Design review of the part built by this model. Coordinates are the model's own, in mm. Face numbers are marked on the shaded views. Round coordinates to 2 decimals unless told otherwise and drop trailing zeros. Order: outer loops, then holes, each group sorted by start corner. A loop starts at its lowest first (then second) coordinate and runs counter-clockwise, first axis right, second up. Notation, with made-up numbers: (17.25, 31) - (51.25, 31) arc R15 ccw to (51.25, 48) - close; hole circle Ø10 at (70, 68). An arc over 180 degrees is marked (long way). Use CSV: the item, a comma, the result in double quotes.
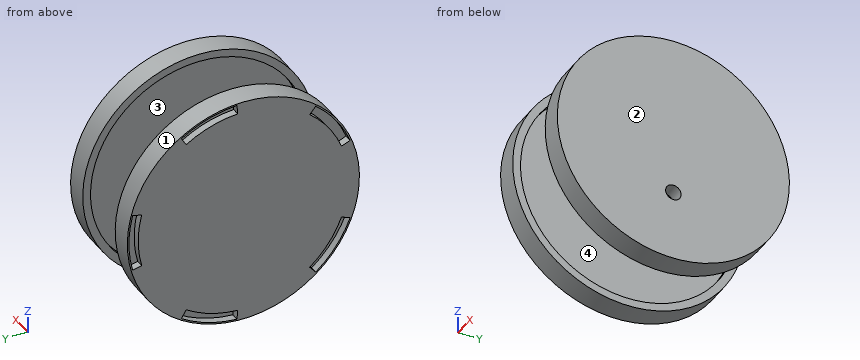
from build123d import *

# Parameters (mm, degrees)
CUT_EXTRUDE1_DEPTH = 5
CIRPATTERN1_COUNT  = 5
SKETCH4_R          = 5
CUT_EXTRUDE4_DEPTH = 16


with BuildPart() as part:
    # Sketch1 → Revolve2 (revolve)
    with BuildSketch(Plane.XY, mode=Mode.PRIVATE) as revolve2_sk:
        Polygon((-52.115384615, 0), (17.884615385, 0), (17.884615385, 75), (2.884615385, 75), (2.884615385, 70), (7.884615385, 70), (7.884615385, 20), (-42.115384615, 20), (-42.115384615, 70), (-37.115384615, 70), (-37.115384615, 75), (-52.115384615, 75), align=None)
    revolve(revolve2_sk.sketch.rotate(Axis((-114.1965821, 0, 0), (1, 0, 0)), 90), axis=Axis((-114.1965821, 0, 0), (1, 0, 0)))

    # Sketch2 → Cut-Extrude1 (cut)
    with BuildSketch(Plane.ZY.offset(52.115384615)):
        with BuildLine():
            Line((-18.889553649, 71.548478411), (-17.514771122, 65.705652668))
            ThreePointArc((-17.514771122, 65.705652668), (0, 68), (17.514771122, 65.705652668))
            Line((17.514771122, 65.705652668), (18.889553649, 71.548478411))
            ThreePointArc((18.889553649, 71.548478411), (0, 74), (-18.889553649, 71.548478411))
        make_face()
    cut_extrude1 = extrude(amount=-CUT_EXTRUDE1_DEPTH, mode=Mode.SUBTRACT)

    # CirPattern1: Cut-Extrude1 ×5 about axis
    cirpattern1_axis = Axis((0, 0, 0), (1, 0, 0))
    for i in range(1, CIRPATTERN1_COUNT):
        add(cut_extrude1.rotate(cirpattern1_axis, i * 360 / CIRPATTERN1_COUNT), mode=Mode.SUBTRACT)

    # Sketch4 → Cut-Extrude4 (cut)
    with BuildSketch(Plane(origin=(17.884615385, 0, 0), x_dir=(0, 0, -1), z_dir=(1, 0, 0))):
        with Locations((29.519700861, 0)):
            Circle(SKETCH4_R)
    extrude(amount=-CUT_EXTRUDE4_DEPTH, mode=Mode.SUBTRACT)


solid = part.part
1) The part is to be moulded in two halves that separate along Z. For the marked faces 1, 2, 3 and 4, say which applies: +Z half, -Z half, draft (parallel to the pull), parting line (faces both ways), or undercut.
Data:
face 1,"parting line"
face 2,"draft"
face 3,"undercut"
face 4,"undercut"
2) We need section C-C (x = 12). Give the boundary of the cut face in (y, z).
Data:
outline,"circle Ø150 at (0, 0); hole circle Ø10 at (0, -29.52)"
3) To check wall thickness, follow L1, parallel to Y at x = -38, z = 0; L2, parallel to X at y = 6, z = -46.5; L3, parallel to X at y = 35, z = -61.5. State the ranges of each line that lie inside material, in increasing order. Write a range as from..to.
Data:
L1,"y = -75..-70, -20..20, 70..75"
L2,"x = -52.12..-42.12, 7.88..17.88"
L3,"x = -47.12..-37.12, 2.88..17.88"
4) We need section D-D (x = -8). Give the boundary of the cut face in (y, z), then the cut area to 3 significant figures.
Data:
outline,"circle Ø40 at (0, 0)"
area,"1,260 mm2"
5) We need section A-A (z = 0). Give the boundary of the cut face in (x, y), then the cut area to 3 significant figures.
Data:
outline,"(-52.12, -75) - (-37.12, -75) - (-37.12, -70) - (-42.12, -70) - (-42.12, -20) - (7.88, -20) - (7.88, -70) - (2.88, -70) - (2.88, -75) - (17.88, -75) - (17.88, 75) - (2.88, 75) - (2.88, 70) - (7.88, 70) - (7.88, 20) - (-42.12, 20) - (-42.12, 70) - (-37.12, 70) - (-37.12, 75) - (-52.12, 75) - (-52.12, 74) - (-47.12, 74) - (-47.12, 68) - (-52.12, 68) - close"
area,"5,070 mm2"
6) Insertion check: pin 1 Ø9 at (y, z) = (0, -29.52) entering from +X; pin 2 Ø4 at (x, z) = (-3.5, 10) entering from +Y; pin 3 Ø1 at (x, z) = (-44.5, 19.5) entering from -Y. Each pin has a flat end and moves straight along its axis. Give the tip position at first contact, or say it passes through.
Data:
pin 1,"stops at x = -42.12"
pin 2,"stops at y = 18.33"
pin 3,"stops at y = -72.55"
7) We need section B-B (y = 0). Give the boundary of the cut face in (x, z), then the cut area to 3 significant figures.
Data:
outline,"(-52.12, -75) - (-37.12, -75) - (-37.12, -70) - (-42.12, -70) - (-42.12, -20) - (7.88, -20) - (7.88, -24.52) - (17.88, -24.52) - (17.88, 75) - (2.88, 75) - (2.88, 70) - (7.88, 70) - (7.88, 20) - (-42.12, 20) - (-42.12, 70) - (-37.12, 70) - (-37.12, 75) - (-52.12, 75) - close; (2.88, -75) - (17.88, -75) - (17.88, -34.52) - (7.88, -34.52) - (7.88, -70) - (2.88, -70) - close"
area,"5,000 mm2"
